Source: three-view drawing plus pictorial views. Frame: mm from the lowest corner of the part. A direction names the side the tool comes from. Give positions to 0.01 mm unless a question says otherwise; leave off trailing zeros. Write each loop counter-clockwise with the first axis right and the second up, starting at its lowest first coordinate (ties: lowest second). Pieces come first, ordered by that corner, then holes.
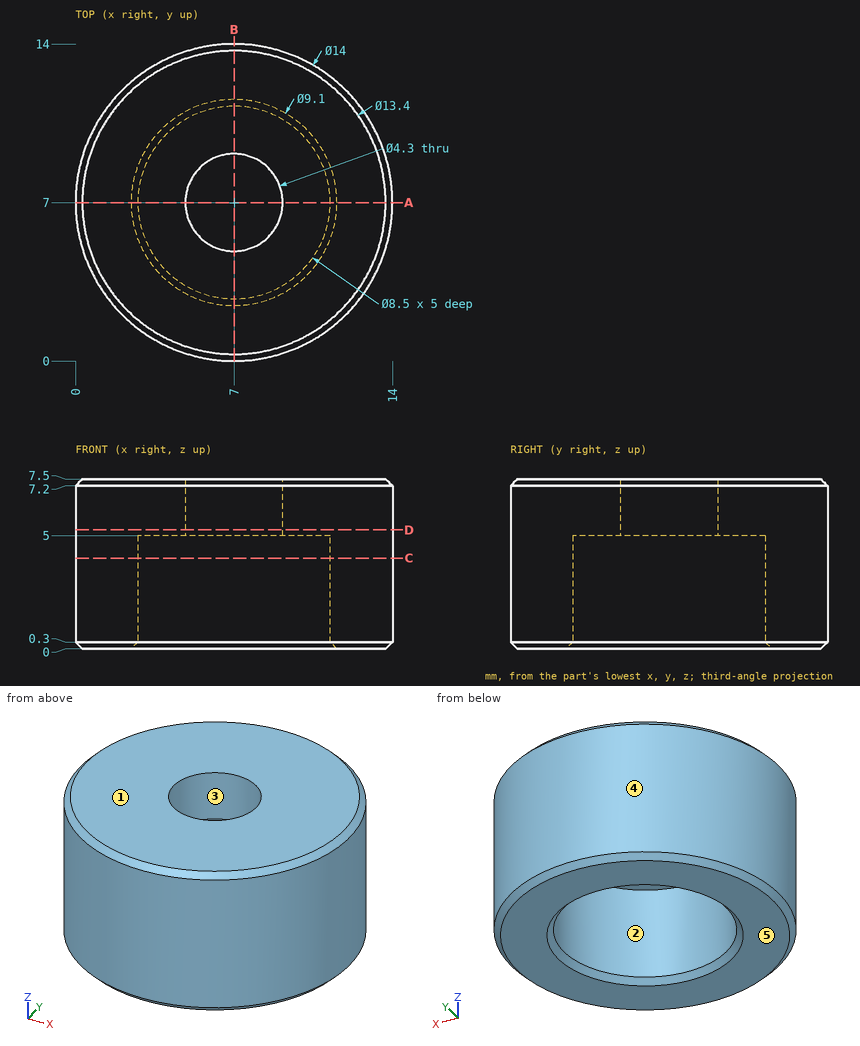
Q1. Section C-C on z = 4. Output: boundary loops of the cut face in (x, y), plus the area to 3 significant figures.
Filled sheet:
outline: circle Ø14 at (7, 7); hole circle Ø8.5 at (7, 7)
area: 97.2 mm2
Q2. Pull-direction query (X, two-part tool) for the marked faces 3, 4 and 5; classes: released by +X, released by -X, zero draft, split by the parting line, or undercut.
Filled sheet:
face 3: undercut
face 4: split by the parting line
face 5: zero draft
Q3. Section A-A on y = 7. Output: boundary loops of the cut face in (x, z), plus the area to 3 significant figures.
Filled sheet:
outline: (0, 0.3) - (0.3, 0) - (2.45, 0) - (2.75, 0.3) - (2.75, 5) - (4.85, 5) - (4.85, 7.5) - (0.3, 7.5) - (0, 7.2) - close; (9.15, 5) - (11.25, 5) - (11.25, 0.3) - (11.55, 0) - (13.7, 0) - (14, 0.3) - (14, 7.2) - (13.7, 7.5) - (9.15, 7.5) - close
area: 51.5 mm2
Q4. Ray query, line 1 along Y through (x, z) = (7, 5.95); line 2 along Y through (x, z) = (7, 2.2); line 3 along Z through (x, y) = (10.25, 9.5). Return the intervals inside material, ascending.
Filled sheet:
line 1: y = 0 to 4.85, 9.15 to 14
line 2: y = 0 to 2.75, 11.25 to 14
line 3: z = 5 to 7.5
Q5. Access query for the marked faces 1 and 2. Directions: +Z, -Z, +X, -X, +Y, -Y. A direction counts if a zero-diameter tool reaches every point of the face in a straight line with its end or side. Return the directions, or none.
Filled sheet:
face 1: +Z, +X, -X, +Y, -Y
face 2: -Z
Q6. Section D-D on z = 5.25. Output: boundary loops of the cut face in (x, y).
Filled sheet:
outline: circle Ø14 at (7, 7); hole circle Ø4.3 at (7, 7)
Q7. Pin query (flat end, axial travel): P1, Ø2, axis at x = 10.5, z = 3.5, coming from the -Y side; P2, Ø1, axis at y = 5.5, z = 2, coming from the -X side; P3, Ø5, axis at x = 3.5, y = 12, coming from the -Z side; P4, Ø2.5, axis at x = 6, y = 8, coming from the -Z side. Return the tip coordinate at first contact, or that it passes through.
Filled sheet:
P1: stops at y = 0.46
P2: stops at x = 0.07
P3: stops at z = 0
P4: stops at z = 5
